from build123d import *

# Parameters (mm, degrees)
SKETCH1_W           = 220
SKETCH1_H           = 140
BOSS_EXTRUDE1_DEPTH = 10
SKETCH2_W           = 220
SKETCH2_H           = 10
BOSS_EXTRUDE2_DEPTH = 30
SKETCH3_W           = 220
SKETCH3_H           = 10
BOSS_EXTRUDE3_DEPTH = 25
SKETCH4_W           = 220
SKETCH4_H           = 10
BOSS_EXTRUDE4_DEPTH = 20


with BuildPart() as part:
    # Sketch1 → Boss-Extrude1 (new body)
    with BuildSketch(Plane(origin=(0, 0, 0), x_dir=(1, 0, 0), z_dir=(0, 1, 0))):
        Rectangle(SKETCH1_W, SKETCH1_H)
    extrude(amount=BOSS_EXTRUDE1_DEPTH)

    # Sketch2 → Boss-Extrude2 (add)
    with BuildSketch(Plane(origin=(0, 10, 0), x_dir=(1, 0, 0), z_dir=(0, 1, 0))):
        with Locations((0, 65)):
            Rectangle(SKETCH2_W, SKETCH2_H)
        with Locations((0, -65)):
            Rectangle(SKETCH2_W, SKETCH2_H)
    extrude(amount=BOSS_EXTRUDE2_DEPTH)

    # Sketch3 → Boss-Extrude3 (add)
    with BuildSketch(Plane.XY.offset(-60)):
        with Locations((0, 35)):
            Rectangle(SKETCH3_W, SKETCH3_H)
    boss_extrude3 = extrude(amount=BOSS_EXTRUDE3_DEPTH)

    # Mirror1: Boss-Extrude3 across plane
    add(boss_extrude3.mirror(Plane.XY))

    # Sketch4 → Boss-Extrude4 (add)
    with BuildSketch(Plane.XZ.offset(-30)):
        with Locations((0, -40)):
            Rectangle(SKETCH4_W, SKETCH4_H)
    boss_extrude4 = extrude(amount=BOSS_EXTRUDE4_DEPTH)

    # Mirror2: Boss-Extrude4 across plane
    add(boss_extrude4.mirror(Plane.XY))


solid = part.part
Source: CAD feature listing. Evaluate the final solid. Frame: model axes, mm. A direction names the side the tool comes from. Give positions to 0.01 mm unless a question says otherwise; leave off trailing zeros. Loops run counter-clockwise (first coordinate to the right, second up) from the corner with the lowest first, then second, coordinate; pieces in that order, holes last. Notation, with made-up numbers: (-4.75, 28.5) -> (15.25, 28.5) arc R10 cw to (15.25, 36.5) -> close; hole circle Ø4 at (-20.5, 49.5). An arc over 180 degrees is marked (long way). Use a Markdown table: item, result. Add a question column.
1) Section query C-C, the plane z = -52.5. Return the cut outline in (x, y), then the cut area to 3 significant figures.
2) Reachability of faces 1 (the face through (110, 7, 1)), 2 (the face through (-2, 25, 35)), 3 (the face through (-2, 20, 45)) from +Z, -Z, +X, -X, +Y, -Y: full face, straight path, thin tool, end or side. Return the list, or none.
3) Section query B-B, the plane x = 79. Return the cut outline in (y, z).
4) Section query A-A, the plane y = 26. Return the cut outline in (x, z), then the cut area to 3 significant figures.
5) Section query D-D, the plane z = 22. Return the cut outline in (x, y), then the cut area to 3 significant figures.
6) First-contact query: pin 1 (8 mm diameter, centred on y = 16.5, z = -27, fed in from -X); pin 2 (4 mm diameter, centred on x = 48.5, z = 17.5, fed in from +Y). Flat tips, straight axial feed; report the tip coordinate or a pass-through.
7) Pull-direction query (Y, two-part tool) for faces 4 (the face through (-2, 40, 53)), 5 (the face through (-2, 20, 70)), 6 (the face through (-2, 10, -53)); classes: +Y half, -Y half, draft (parallel to the pull), parting line (faces both ways), or undercut.
8) Line query: line 1 along Z through (x, y) = (-75.5, 14); line 2 along Z through (x, y) = (68.5, 32); line 3 along Y through (x, z) = (24, 50). Output: solid intervals per line, ascending. Write a range as [from, to].
Numbers:
| question | item | result |
|---|---|---|
| 1 | outline | (-110, 0) -> (110, 0) -> (110, 10) -> (-110, 10) -> close; (-110, 30) -> (110, 30) -> (110, 40) -> (-110, 40) -> close |
| 1 | area | 4,400 mm2 |
| 2 | face 1 | +Z, -Z, +X, +Y, -Y |
| 2 | face 2 | +X, -X, +Y |
| 2 | face 3 | +X, -X |
| 3 | outline | (0, -70) -> (40, -70) -> (40, -35) -> (10, -35) -> (10, 35) -> (40, 35) -> (40, 70) -> (0, 70) -> close; hole (10, -60) -> (30, -60) -> (30, -45) -> (10, -45) -> close; hole (10, 45) -> (30, 45) -> (30, 60) -> (10, 60) -> close |
| 4 | outline | (-110, -70) -> (110, -70) -> (110, -60) -> (-110, -60) -> close; (-110, -45) -> (110, -45) -> (110, -35) -> (-110, -35) -> close; (-110, 35) -> (110, 35) -> (110, 45) -> (-110, 45) -> close; (-110, 60) -> (110, 60) -> (110, 70) -> (-110, 70) -> close |
| 4 | area | 8,800 mm2 |
| 5 | outline | (-110, 0) -> (110, 0) -> (110, 10) -> (-110, 10) -> close |
| 5 | area | 2,200 mm2 |
| 6 | pin 1 | passes through |
| 6 | pin 2 | stops at y = 10 |
| 7 | face 4 | +Y half |
| 7 | face 5 | draft |
| 7 | face 6 | undercut |
| 8 | line 1 | z = [-70, -60], [-45, -35], [35, 45], [60, 70] |
| 8 | line 2 | z = [-70, -35], [35, 70] |
| 8 | line 3 | y = [0, 10], [30, 40] |
